Can you work these out from the drawing? Everything is in mm from the part's minimum corner. A direction names the side the tool comes from. Round coordinates to 2 decimals unless told otherwise and drop trailing zeros. Loops run counter-clockwise (first coordinate to the right, second up) from the corner with the lowest first, then second, coordinate; pieces in that order, holes last. Notation, with made-up numbers: (-16.75, 4.25) -> (-2.75, 4.25) arc R8 cw to (-2.75, 17.25) -> close; hole circle Ø8 at (77.25, -16.75). An arc over 180 degrees is marked (long way). One line per item, written item: value.
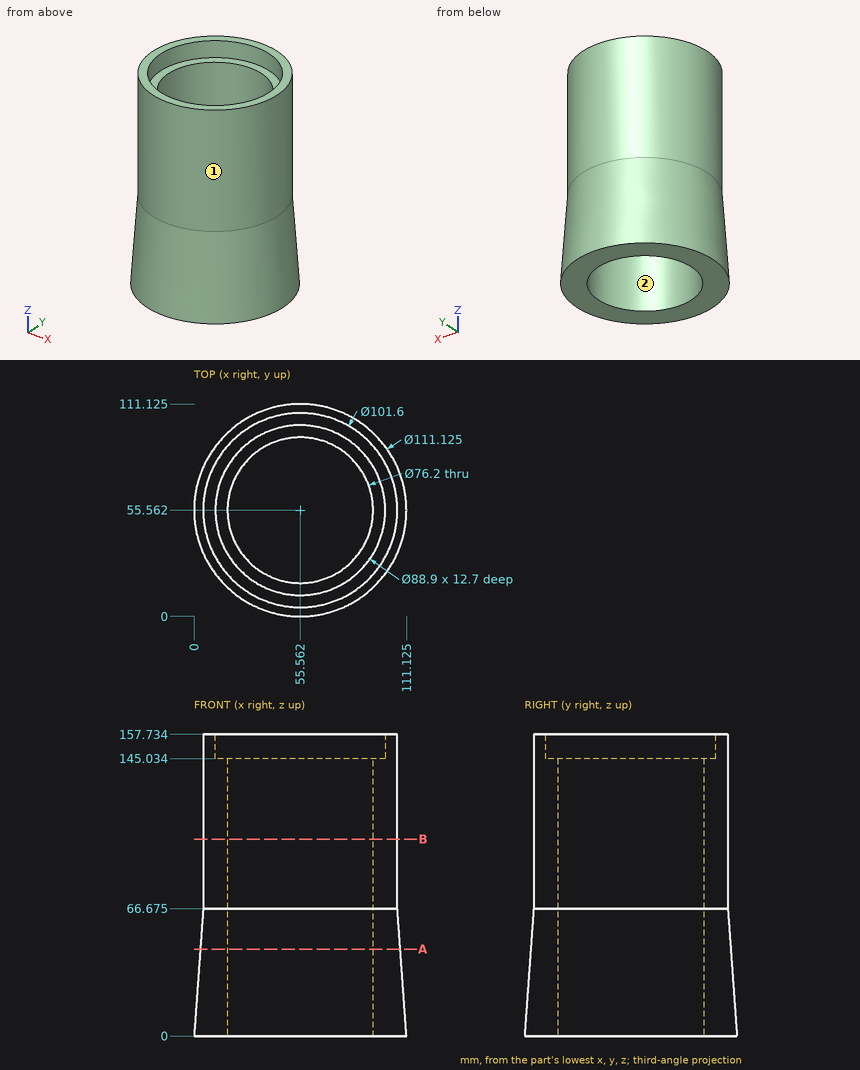
(1) Imagine slicing it at A-A on z = 45.5. Write out the boundary of the cut face in (x, y) (1 decimal).
Results below:
outline: circle Ø104.6 at (55.6, 55.6); hole circle Ø76.2 at (55.6, 55.6)
(2) On a 3-axis mill with a long thin cutter (end or side, diameter ignored), from which of +Z, -Z, +X, -X, +Y, -Y can I reach the whole of each face in a straight line? I mean the marked faces 1 and 2. Say none if no direction works.
Results below:
face 1: +Z
face 2: +Z, -Z
(3) Imagine slicing it at B-B on z = 103. Write out the boundary of the cut face in (x, y).
Results below:
outline: circle Ø101.6 at (55.56, 55.56); hole circle Ø76.2 at (55.56, 55.56)
(4) Please list where these lines run through material, in increasing order: L1, parallel to X at y = 67, z = 40 (1 decimal); L2, parallel to Y at x = 89, z = 55 (1 decimal); L3, parallel to Z at x = 19.5, y = 73.5 (1 decimal).
Results below:
L1: x = 4.1 to 19.2, 91.9 to 107
L2: y = 16.2 to 37.3, 73.8 to 94.9
L3: z = 0 to 145
(5) For pin 1 Ø5 at (x, z) = (66.5, 56) entering from -Y; pin 2 Ø12 at (y, z) = (76.5, 57) entering from +X; pin 3 Ø5 at (x, z) = (57.5, 71) entering from -Y; pin 4 Ø6 at (x, y) = (79, 85) entering from -Z, each with a flat end and sliding along its axis, tell me the tip position at first contact or that it passes through.
Results below:
pin 1: stops at y = 4.66
pin 2: stops at x = 104.89
pin 3: stops at y = 4.76
pin 4: stops at z = 0
